Verification items for the finished model (mm, model axes). Face numbers are marked on the shaded views. Give positions to 0.01 mm unless a question says otherwise; leave off trailing zeros. Write each loop counter-clockwise with the first axis right and the second up, starting at its lowest first coordinate (ties: lowest second). Pieces come first, ordered by that corner, then holes.
Autodesk Inventor part; units mm, degrees
ref_plane "YZ Plane" through (0, 0, 0) normal (1, 0, 0) x (0, 1, 0)
ref_plane "XZ Plane" through (0, 0, 0) normal (0, 1, 0) x (-1, 0, 0)
ref_plane "XY Plane" through (0, 0, 0) normal (0, 0, 1) x (1, 0, 0)
sketch "Boceto1" plane through (0, 0, 0) normal (0, 1, 0) x (-1, 0, 0)
  circle A0 centre (0, 0) radius 34.5
  circle A1 centre (0, 0) radius 35
  dimension "d0" = 69
  dimension "d1" = 70
extrude "Extrusión1" add sketch "Boceto1" along normal blind 1 contours A0 | A1
sketch "Boceto2" plane through (0, 1, 0) normal (0, 1, 0) x (1, 0, 0)
  circle A0 centre (0, 0) radius 34.5
  circle A1 centre (0, 0) radius 34.75
  dimension "d4" = 69
  dimension "d5" = 69.5
extrude "Extrusión2" add sketch "Boceto2" along normal blind 25
sketch "Boceto3" plane through (0, 1, 0) normal (0, 1, 0) x (1, 0, 0)
  circle A0 centre (0, 0) radius 2.1
  circle A1 centre (0, 0) radius 1.75
  dimension "d8" = 4.2
  dimension "d9" = 3.5
extrude "Extrusión3" add sketch "Boceto3" along normal blind 3
sketch "Boceto4" plane through (0, 1, 0) normal (0, 1, 0) x (1, 0, 0)
  circle A0 centre (0, 0) radius 1.75
  dimension "d14" = 3.5
extrude "Extrusión4" cut sketch "Boceto4" against normal through all
sketch "Boceto5" plane through (0, 26, 0) normal (0, 1, 0) x (1, 0, 0)
  circle A0 centre (0, 0) radius 35
  circle A1 centre (0, 0) radius 1.75
  circle A2 centre (0, 0) radius 34.75
  dimension "d15" = 69.5
  dimension "d16" = 70
extrude "Extrusión5" cut sketch "Boceto5" against normal through all
properties part number "Molde_V002"
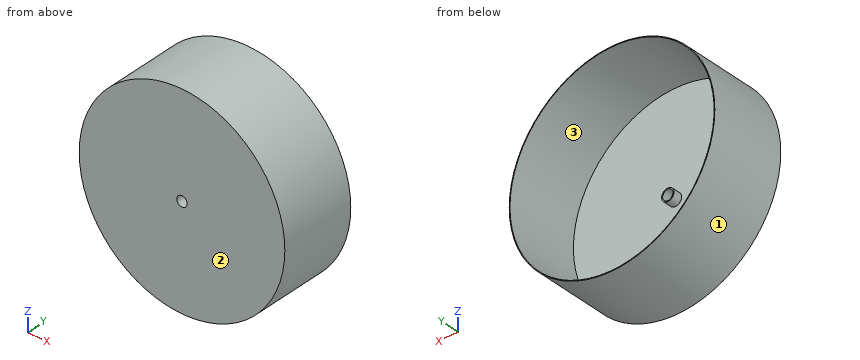
Item 1: Release check for a two-part mould opening along Z. For the marked faces 1, 2 and 3 record: released by +Z, released by -Z, zero draft, split by the parting line, or undercut.
Answer key:
face 1: split by the parting line
face 2: zero draft
face 3: undercut
Item 2: Sectioned sample at A-A on z = 0. Record the cut outline in (x, y), then the cut area to 3 significant figures.
Answer key:
outline: (-34.75, 0) - (-1.75, 0) - (-1.75, 4) - (-2.1, 4) - (-2.1, 1) - (-34.5, 1) - (-34.5, 26) - (-34.75, 26) - close; (1.75, 0) - (34.75, 0) - (34.75, 26) - (34.5, 26) - (34.5, 1) - (2.1, 1) - (2.1, 4) - (1.75, 4) - close
area: 80.6 mm2
Item 3: Sectioned sample at D-D on z = 27. Record the cut outline in (x, y).
Answer key:
outline: (-21.88, 0) - (21.88, 0) - (21.88, 26) - (21.48, 26) - (21.48, 1) - (-21.48, 1) - (-21.48, 26) - (-21.88, 26) - close
Item 4: Depth check by flat-ended pin: pin 1 (20.5 mm diameter, centred on x = 4, z = 8, fed in from +Y); pin 2 (10 mm diameter, centred on x = 8, y = 7, fed in from +Z); pin 3 (10 mm diameter, centred on x = 13.5, y = 12.5, fed in from +Z). Enter the tip coordinate at first touch or a pass-through.
Answer key:
pin 1: stops at y = 4
pin 2: stops at z = 34.62
pin 3: stops at z = 33.69
Item 5: Scan lines: line 1 along X through (y, z) = (3.05, 0); line 2 along Z through (x, y) = (0, 12.25); line 3 along Y through (x, z) = (-3, 4). Record each from-to range of solid material in increasing order.
Answer key:
line 1: x = -34.75 to -34.5, -2.1 to -1.75, 1.75 to 2.1, 34.5 to 34.75
line 2: z = -34.75 to -34.5, 34.5 to 34.75
line 3: y = 0 to 1
Item 6: Sectioned sample at C-C on y = 12. Record the cut outline in (x, z).
Answer key:
outline: circle Ø69.5 at (0, 0); hole circle Ø69 at (0, 0)
Item 7: Sectioned sample at B-B on x = 0. Record the cut outline in (y, z), then the cut area to 3 significant figures.
Answer key:
outline: (0, -34.75) - (26, -34.75) - (26, -34.5) - (1, -34.5) - (1, -2.1) - (4, -2.1) - (4, -1.75) - (0, -1.75) - close; (0, 1.75) - (4, 1.75) - (4, 2.1) - (1, 2.1) - (1, 34.5) - (26, 34.5) - (26, 34.75) - (0, 34.75) - close
area: 80.6 mm2
